The listing builds one solid part. Answer for the finished solid, in the listing's coordinates (mm). A direction names the side the tool comes from. Round coordinates to 2 decimals unless told otherwise and drop trailing zeros. Order: outer loops, then holes, each group sorted by start corner. A loop starts at its lowest first (then second) coordinate and runs counter-clockwise, first axis right, second up. Notation, with made-up numbers: M 81,78 L 127,78 A25 ccw 127,104 Z; hole C 22,87.25 d11. An arc over 180 degrees is marked long. Put each result on its own line as item: value. Start each with the question number.
1. The part is cut by section C-C (y = 1.5). Give the vertices of the cut face in (x, z).
2. Consider line 1 (Y direction, x = -5.5, z = -8.5); line 2 (X direction, y = -22.5, z = -4.75); line 3 (X direction, y = -3.5, z = -11.5). Determine where each line is inside the solid, lowest interval first.
3. The mould has two halves that part along Z. Classify faces 5 (the face through (-3, -10, 7.62)), 6 (the face through (-81.28, 3, -6)), 7 (the face through (-41, 3, 0)), 8 (the face through (-39.37, 3, -8)): +Z half, -Z half, draft (parallel to the pull), parting line (faces both ways), or undercut.
4. Each of these flat-tipped pins is pushed along its axis until it touches: pin 1 Ø12 at (x, y) = (-38, -1) entering from +Z; pin 2 Ø4 at (x, y) = (-41.5, -1) entering from -Z; pin 3 Ø3 at (y, z) = (-21, -9) entering from -X; pin 4 Ø1 at (y, z) = (-7, 2.5) entering from +X. Where does it stop, or does it pass through?
5. The part is cut by section B-B (x = -74). Give the vertices of the cut face in (y, z), then the cut area to 3 significant figures.
6. The part is cut by section A-A (z = -14.5). Give the vertices of the cut face in (x, y), then the cut area to 3 significant figures.
7. Which of the six approach directions +Z, -Z, +X, -X, +Y, -Y give full straight-line access (tool end or side, diameter ignored) to faces 1 (the face through (-41, 7, -12.7)), 2 (the face through (0, -13, -6)), 3 (the face through (-5.068, -1, 6)), 4 (the face through (-3, -4, 3.81))?
8. The part is cut by section D-D (x = -41). Give the vertices of the cut face in (y, z) (3 decimals).
from build123d import *

# Parameters (mm, degrees)
SKETCH1_W           = 81.28
SKETCH1_H           = 5.08
BOSS_EXTRUDE1_DEPTH = 3.81
SKETCH3_W           = 5.067533081
SKETCH3_H           = 3.81
BOSS_EXTRUDE2_DEPTH = 30.48
SKETCH4_W           = 26.67
SKETCH4_H           = 17.78
BOSS_EXTRUDE3_DEPTH = 6.35
SKETCH6_W           = 20.32
SKETCH6_H           = 5.08
BOSS_EXTRUDE4_DEPTH = 3.81
SKETCH7_W           = 4.626355507
SKETCH7_H           = 5.08
BOSS_EXTRUDE5_DEPTH = 38.1
SKETCH8_W           = 13.97
SKETCH8_H           = 13.97
BOSS_EXTRUDE6_DEPTH = 3.81
SKETCH9_W           = 3.81
SKETCH9_H           = 4.445
CUT_EXTRUDE1_DEPTH  = 56.663101782
FILLET1_R           = 7.62


with BuildPart() as part:
    # Sketch1 → Boss-Extrude1 (new body)
    with BuildSketch(Plane.XY):
        with Locations((-40.64, 2.54)):
            Rectangle(SKETCH1_W, SKETCH1_H)
    extrude(amount=BOSS_EXTRUDE1_DEPTH)

    # Sketch3 → Boss-Extrude2 (add)
    with BuildSketch(Plane(origin=(0, 5.08, 0), x_dir=(1, 0, 0), z_dir=(0, 1, 0))):
        with Locations((-2.533766541, -5.715)):
            Rectangle(SKETCH3_W, SKETCH3_H)
    extrude(amount=-BOSS_EXTRUDE2_DEPTH)

    # Sketch4 → Boss-Extrude3 (add)
    with BuildSketch(Plane(origin=(0, 0, 0), x_dir=(0, 0, -1), z_dir=(1, 0, 0))):
        with Locations((5.715, -16.51)):
            Rectangle(SKETCH4_W, SKETCH4_H)
    extrude(amount=-BOSS_EXTRUDE3_DEPTH)

    # Sketch6 → Boss-Extrude4 (add)
    with BuildSketch(Plane.ZY.offset(81.28)):
        with Locations((-6.35, 2.54)):
            Rectangle(SKETCH6_W, SKETCH6_H)
    extrude(amount=BOSS_EXTRUDE4_DEPTH)

    # Sketch7 → Boss-Extrude5 (add)
    with BuildSketch(Plane(origin=(-81.28, 0, 0), x_dir=(0, 0, -1), z_dir=(1, 0, 0))):
        with Locations((14.196822247, 2.54)):
            Rectangle(SKETCH7_W, SKETCH7_H)
    extrude(amount=BOSS_EXTRUDE5_DEPTH)

    # Sketch8 → Boss-Extrude6 (add)
    with BuildSketch(Plane(origin=(-43.18, 0, 0), x_dir=(0, 0, -1), z_dir=(1, 0, 0))):
        with Locations((9.525, 2.54)):
            Rectangle(SKETCH8_W, SKETCH8_H)
    extrude(amount=BOSS_EXTRUDE6_DEPTH)

    # Sketch9 → Cut-Extrude1 (cut, through all)
    with BuildSketch(Plane(origin=(-39.37, 0, 0), x_dir=(0, 0, -1), z_dir=(1, 0, 0))):
        with Locations((14.605, -2.2225)):
            Rectangle(SKETCH9_W, SKETCH9_H)
        with Locations((14.605, 7.3025)):
            Rectangle(SKETCH9_W, SKETCH9_H)
    extrude(amount=-CUT_EXTRUDE1_DEPTH, mode=Mode.SUBTRACT)

    # Fillet1
    fillet1_edges = [part.edges().sort_by_distance(p)[0] for p in [
        (-43.18, 2.54, -11.883644493),
    ]]
    fillet(fillet1_edges, radius=FILLET1_R)


solid = part.part
Resolved:
1. outline: M -85.09,-16.51 L -39.37,-16.51 L -39.37,-2.54 L -43.18,-2.54 L -43.18,-4.26 A7.62 cw -50.8,-11.88 L -81.28,-11.88 L -81.28,0 L 0,0 L 0,7.62 L -5.07,7.62 L -5.07,3.81 L -85.09,3.81 Z
2. line 1: -25.4 to -7.62
2. line 2: -6.35 to 0
2. line 3: -43.18 to -39.37
3. face 5: +Z half
3. face 6: undercut
3. face 7: undercut
3. face 8: draft
4. pin 1: z = 3.81
4. pin 2: z = -16.51
4. pin 3: x = -6.35
4. pin 4: through
5. outline: M 0,-16.51 L 5.08,-16.51 L 5.08,-11.88 L 0,-11.88 Z; M 0,0 L 5.08,0 L 5.08,3.81 L 0,3.81 Z
5. area: 42.9 mm2
6. outline: M -85.09,0 L -39.37,0 L -39.37,5.08 L -85.09,5.08 Z; M -6.35,-25.4 L 0,-25.4 L 0,-7.62 L -6.35,-7.62 Z
6. area: 345 mm2
7. face 1: -Z, +X, -X, +Y
7. face 2: +Z, -Z, +X, +Y, -Y
7. face 3: +Z, -X, +Y
7. face 4: -Z, +X, -X
8. outline: M -4.445,-12.7 L 0,-12.7 L 0,-16.51 L 5.08,-16.51 L 5.08,-12.7 L 9.525,-12.7 L 9.525,-2.54 L -4.445,-2.54 Z; M 0,0 L 5.08,0 L 5.08,3.81 L 0,3.81 Z
